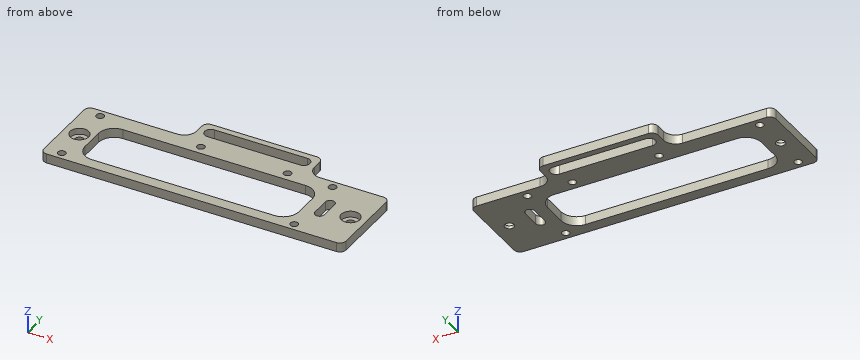
```python
from build123d import *

# Parameters (mm, degrees)
SKETCH_3_W               = 97.5
SKETCH_3_H               = 27
EXTRUDE_1_DEPTH          = 3
SKETCH_4_R               = 1.25
CUT_EXTRUDE_1_DEPTH      = 51.673587795
SKETCH_7_W               = 4
SKETCH_7_H               = 8
EXTRUDE_2_DEPTH          = 5
SKETCH_8_W               = 38
SKETCH_8_H               = 9
EXTRUDE_3_DEPTH          = 3
FILLET_3_R               = 4
FILLET_4_R               = 2
CUT_EXTRUDE_4_DEPTH      = 55.284551209
CUT_EXTRUDE_4_DEPTH_BACK = 5
SKETCH_9_W               = 4
SKETCH_9_H               = 8
SKETCH_13_R              = 1.5
CUT_EXTRUDE_7_DEPTH      = 54.775575311
CUT_EXTRUDE_8_DEPTH      = 54.775575311
SKETCH_16_R              = 3
CUT_EXTRUDE_9_DEPTH      = 2
CUT_EXTRUDE_10_DEPTH     = 10
FILLET_5_R               = 5
FILLET_6_R               = 2


with BuildPart() as part:
    # 草图3 → 凸台-拉伸1 (new body)
    with BuildSketch(Plane.XY):
        Rectangle(SKETCH_3_W, SKETCH_3_H)
    extrude(amount=EXTRUDE_1_DEPTH)

    # 草图4 → 切除-拉伸1 (cut, through all)
    with BuildSketch(Plane.XY.offset(3)):
        with Locations((-43.25, 11)):
            Circle(SKETCH_4_R)
        with Locations((-43.25, -11)):
            Circle(SKETCH_4_R)
        with Locations((31.75, 11)):
            Circle(SKETCH_4_R)
        with Locations((31.75, -11)):
            Circle(SKETCH_4_R)
        with Locations((17.25, 11)):
            Circle(SKETCH_4_R)
        with Locations((-10.75, 11)):
            Circle(SKETCH_4_R)
    extrude(amount=-CUT_EXTRUDE_1_DEPTH, mode=Mode.SUBTRACT)

    # 草图7 → 凸台-拉伸2 (add)
    with BuildSketch(Plane(origin=(0, 0, 0), x_dir=(-1, 0, 0), z_dir=(0, 0, -1))):
        with Locations((46.75, 0.5)):
            Rectangle(SKETCH_7_W, SKETCH_7_H)
        with Locations((-46.75, 0.5)):
            Rectangle(SKETCH_7_W, SKETCH_7_H)
    extrude(amount=EXTRUDE_2_DEPTH)

    # 草图8 → 凸台-拉伸3 (add)
    with BuildSketch(Plane.XY.offset(3)):
        with Locations((3.25, 18)):
            Rectangle(SKETCH_8_W, SKETCH_8_H)
        with BuildLine():
            Line((-11.75, 20.5), (18.25, 20.5))
            ThreePointArc((18.25, 20.5), (20.25, 18.5), (18.25, 16.5))
            Line((18.25, 16.5), (-11.75, 16.5))
            ThreePointArc((-11.75, 16.5), (-13.75, 18.5), (-11.75, 20.5))
        make_face(mode=Mode.SUBTRACT)
    extrude(amount=-EXTRUDE_3_DEPTH)

    # 圆角3
    fillet_3_edges = [part.edges().sort_by_distance(p)[0] for p in [
        (22.25, 13.5, 1.5),
        (-15.75, 13.5, 1.5),
    ]]
    fillet(fillet_3_edges, radius=FILLET_3_R)

    # 圆角4
    fillet_4_edges = [part.edges().sort_by_distance(p)[0] for p in [
        (22.25, 22.5, 1.5),
        (-15.75, 22.5, 1.5),
    ]]
    fillet(fillet_4_edges, radius=FILLET_4_R)

    # 草图9 → 切除-拉伸4 (cut, two sides: drawn at the far end of the back side and taken through both)
    with BuildSketch(Plane(origin=(0, 0, -5), x_dir=(-1, 0, 0), z_dir=(0, 0, -1)).offset(-CUT_EXTRUDE_4_DEPTH_BACK)):
        with Locations((-46.75, 0.5)):
            Rectangle(SKETCH_9_W, SKETCH_9_H)
        with Locations((46.75, 0.5)):
            Rectangle(SKETCH_9_W, SKETCH_9_H)
    extrude(amount=CUT_EXTRUDE_4_DEPTH + CUT_EXTRUDE_4_DEPTH_BACK, mode=Mode.SUBTRACT)

    # 草图13 → 切除-拉伸7 (cut, through all)
    with BuildSketch(Plane(origin=(0, 0, 0), x_dir=(-1, 0, 0), z_dir=(0, 0, -1))):
        with Locations((-43.75, 0)):
            Circle(SKETCH_13_R)
        with Locations((43.75, 0)):
            Circle(SKETCH_13_R)
    extrude(amount=-CUT_EXTRUDE_7_DEPTH, mode=Mode.SUBTRACT)

    # 草图14 → 切除-拉伸8 (cut, through all)
    with BuildSketch(Plane.XY.offset(3)):
        with BuildLine():
            Line((36.75, 3.35), (36.75, -2.65))
            ThreePointArc((36.75, -2.65), (35.25, -4.15), (33.75, -2.65))
            Line((33.75, -2.65), (33.75, 3.35))
            ThreePointArc((33.75, 3.35), (35.25, 4.85), (36.75, 3.35))
        make_face()
    extrude(amount=-CUT_EXTRUDE_8_DEPTH, mode=Mode.SUBTRACT)

    # 草图16 → 切除-拉伸9 (cut)
    with BuildSketch(Plane.XY.offset(3)):
        with Locations((-43.75, 0)):
            Circle(SKETCH_16_R)
        with Locations((43.75, 0)):
            Circle(SKETCH_16_R)
    extrude(amount=-CUT_EXTRUDE_9_DEPTH, mode=Mode.SUBTRACT)

    # 草图17 → 切除-拉伸10 (cut)
    with BuildSketch(Plane(origin=(0, 0, 0), x_dir=(-1, 0, 0), z_dir=(0, 0, -1))):
        Polygon((39.25, -8), (39.25, 8), (-27.75, 8), (-29.75, 8), (-29.75, -9.826666667), (-27.75, -9.826666667), (39.25, -9.826666667), align=None)
    extrude(amount=-CUT_EXTRUDE_10_DEPTH, mode=Mode.SUBTRACT)

    # 圆角5
    fillet_5_edges = [part.edges().sort_by_distance(p)[0] for p in [
        (29.75, 8, 1.5),
        (-39.25, 8, 1.5),
        (-39.25, -9.826666667, 1.5),
        (29.75, -9.826666667, 1.5),
    ]]
    fillet(fillet_5_edges, radius=FILLET_5_R)

    # 圆角6
    fillet_6_edges = [part.edges().sort_by_distance(p)[0] for p in [
        (48.75, -13.5, 1.5),
        (-48.75, -13.5, 1.5),
        (-48.75, 13.5, 1.5),
        (48.75, 13.5, 1.5),
    ]]
    fillet(fillet_6_edges, radius=FILLET_6_R)


solid = part.part
```
Geometry: final body of the model. Coordinates: model frame, mm. Round coordinates to 2 decimals unless told otherwise and drop trailing zeros. Write each loop counter-clockwise with the first axis right and the second up, starting at its lowest first coordinate (ties: lowest second). Pieces come first, ordered by that corner, then holes. Notation, with made-up numbers: (4.25, 5.5) -> (57.25, 5.5) arc R20 ccw to (57.25, 20.5) -> close; hole circle Ø8 at (2, -9). An arc over 180 degrees is marked (long way). Return JSON: item names as keys, results as strings.
Q1. First-contact query: pin 1 Ø3 at (x, y) = (-30.5, 12.5) entering from -Z; pin 2 Ø2.5 at (x, y) = (-43.75, 0) entering from -Z; pin 3 Ø1.5 at (x, z) = (35, 1) entering from +Y; pin 4 Ø1.8 at (x, y) = (44, -1.5) entering from +Z. Flat tips, straight axial feed; report the tip coordinate or a pass-through.
From the geometry:
{"pin 1": "z = 0", "pin 2": "through", "pin 3": "y = 13.5", "pin 4": "z = 1"}
Q2. Section A-A on y = 18.5. Return the cut outline in (x, z), and give its area (3 significant figures).
From the geometry:
{"outline": "(-15.75, 0) -> (-13.75, 0) -> (-13.75, 3) -> (-15.75, 3) -> close; (20.25, 0) -> (22.25, 0) -> (22.25, 3) -> (20.25, 3) -> close", "area": "12.0 mm2"}
Q3. Section B-B on x = -31.5. Return the cut outline in (y, z).
From the geometry:
{"outline": "(-13.5, 0) -> (-9.83, 0) -> (-9.83, 3) -> (-13.5, 3) -> close; (8, 0) -> (13.5, 0) -> (13.5, 3) -> (8, 3) -> close"}
Q4. Section C-C on y = 0. Return the cut outline in (x, z).
From the geometry:
{"outline": "(-48.75, 0) -> (-45.25, 0) -> (-45.25, 1) -> (-46.75, 1) -> (-46.75, 3) -> (-48.75, 3) -> close; (-42.25, 0) -> (-39.25, 0) -> (-39.25, 3) -> (-40.75, 3) -> (-40.75, 1) -> (-42.25, 1) -> close; (29.75, 0) -> (33.75, 0) -> (33.75, 3) -> (29.75, 3) -> close; (36.75, 0) -> (42.25, 0) -> (42.25, 1) -> (40.75, 1) -> (40.75, 3) -> (36.75, 3) -> close; (45.25, 0) -> (48.75, 0) -> (48.75, 3) -> (46.75, 3) -> (46.75, 1) -> (45.25, 1) -> close"}
Q5. Ray query, line 1 (Y direction, x = -10.75, z = 2.2); line 2 (Y direction, x = 2, z = 0.8); line 3 (X direction, y = -10, z = 0.85). Return the intervals inside material, ascending.
From the geometry:
{"line 1": "-13.5 to -9.83, 8 to 9.75, 12.25 to 16.5, 20.5 to 22.5", "line 2": "-13.5 to -9.83, 8 to 16.5, 20.5 to 22.5", "line 3": "-48.75 to -44, -42.5 to 31, 32.5 to 48.75"}
Q6. Section D-D on x = -10.75. Return the cut outline in (y, z), and give its area (3 significant figures).
From the geometry:
{"outline": "(-13.5, 0) -> (-9.83, 0) -> (-9.83, 3) -> (-13.5, 3) -> close; (8, 0) -> (9.75, 0) -> (9.75, 3) -> (8, 3) -> close; (12.25, 0) -> (16.5, 0) -> (16.5, 3) -> (12.25, 3) -> close; (20.5, 0) -> (22.5, 0) -> (22.5, 3) -> (20.5, 3) -> close", "area": "35.0 mm2"}
